Work out the finished part from the listing and answer in its coordinate system (mm). Face numbers are marked on the shaded views. A direction names the side the tool comes from. Coordinates: 2 decimals unless noted, no trailing zeros. Order: outer loops, then holes, each group sorted by start corner. A loop starts at its lowest first (then second) coordinate and runs counter-clockwise, first axis right, second up. Notation, with made-up numbers: (24.5, -13) -> (68.5, -13) arc R21 ccw to (68.5, 4) -> close; hole circle Ø3 at (-5.75, -31.75). An arc over 180 degrees is marked (long way). Use one line per item in the form item = value.
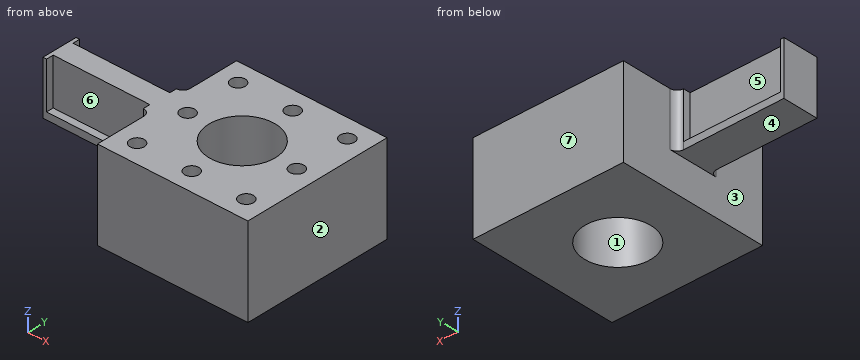
from build123d import *

# Parameters (mm, degrees)
SKETCH_1_W          = 42
SKETCH_1_H          = 42
EXTRUDE_1_DEPTH     = 25
SKETCH_2_R          = 9.25
CUT_EXTRUDE_1_DEPTH = 65.443773943
SKETCH_3_R          = 2
CUT_EXTRUDE_2_DEPTH = 3
EXTRUDE_2_DEPTH     = 30
SKETCH_5_W          = 27
SKETCH_5_H          = 13
CUT_EXTRUDE_3_DEPTH = 2
SKETCH_6_W          = 27
SKETCH_6_H          = 13
CUT_EXTRUDE_4_DEPTH = 2
FILLET_1_R          = 2


with BuildPart() as part:
    # 스케치1 → 보스-돌출1 (new body)
    with BuildSketch(Plane.XY):
        with Locations((21, -21)):
            Rectangle(SKETCH_1_W, SKETCH_1_H)
    extrude(amount=EXTRUDE_1_DEPTH)

    # 스케치2 → 컷-돌출1 (cut, through all)
    with BuildSketch(Plane.XY.offset(25)):
        with Locations((21, -21)):
            Circle(SKETCH_2_R)
    extrude(amount=-CUT_EXTRUDE_1_DEPTH, mode=Mode.SUBTRACT)

    # 스케치3 → 컷-돌출2 (cut)
    with BuildSketch(Plane.XY.offset(25)):
        with Locations((36.25, -36.25)):
            Circle(SKETCH_3_R)
        with Locations((5.75, -36.25)):
            Circle(SKETCH_3_R)
        with Locations((36.25, -5.75)):
            Circle(SKETCH_3_R)
        with Locations((5.75, -5.75)):
            Circle(SKETCH_3_R)
        with Locations((36.25, -21)):
            Circle(SKETCH_3_R)
        with Locations((21, -5.75)):
            Circle(SKETCH_3_R)
        with Locations((21, -36.25)):
            Circle(SKETCH_3_R)
        with Locations((5.75, -21)):
            Circle(SKETCH_3_R)
    extrude(amount=-CUT_EXTRUDE_2_DEPTH, mode=Mode.SUBTRACT)

    # 스케치4 → 보스-돌출2 (add)
    with BuildSketch(Plane.ZY):
        Polygon((25, -21), (25, -26), (10, -26), (10, -16), (25, -16), align=None)
    extrude(amount=EXTRUDE_2_DEPTH)

    # 스케치5 → 컷-돌출3 (cut)
    with BuildSketch(Plane(origin=(0, -26, 0), x_dir=(-1, 0, 0), z_dir=(0, -1, 0))):
        with Locations((15.5, -18.5)):
            Rectangle(SKETCH_5_W, SKETCH_5_H)
    extrude(amount=-CUT_EXTRUDE_3_DEPTH, mode=Mode.SUBTRACT)

    # 스케치6 → 컷-돌출4 (cut)
    with BuildSketch(Plane(origin=(0, -16, 0), x_dir=(1, 0, 0), z_dir=(0, 1, 0))):
        with Locations((-15.5, -18.5)):
            Rectangle(SKETCH_6_W, SKETCH_6_H)
    extrude(amount=-CUT_EXTRUDE_4_DEPTH, mode=Mode.SUBTRACT)

    # 필렛1
    fillet_1_edges = [part.edges().sort_by_distance(p)[0] for p in [
        (0, -16, 17.5),
        (0, -26, 17.5),
    ]]
    fillet(fillet_1_edges, radius=FILLET_1_R)


solid = part.part
(1) The mould has two halves that part along X. Classify the marked faces 1, 2 and 3: released by +X, released by -X, zero draft, split by the parting line, or undercut.
Data:
face_1 = undercut
face_2 = released by +X
face_3 = released by -X
(2) Section C-C on y = -5.75 is taken. Write down the section's boundary in (x, z), plus the area to 3 significant figures.
Data:
outline = (0, 0) -> (42, 0) -> (42, 25) -> (38.25, 25) -> (38.25, 22) -> (34.25, 22) -> (34.25, 25) -> (23, 25) -> (23, 22) -> (19, 22) -> (19, 25) -> (7.75, 25) -> (7.75, 22) -> (3.75, 22) -> (3.75, 25) -> (0, 25) -> close
area = 1,010 mm²
(3) Section B-B on x = 12.5 is taken. Write down the section's boundary in (y, z).
Data:
outline = (-42, 0) -> (-24.65, 0) -> (-24.65, 25) -> (-42, 25) -> close; (-17.35, 0) -> (0, 0) -> (0, 25) -> (-17.35, 25) -> close
(4) Each of these flat-tipped pins is pushed along its axis until it touches: P1, Ø7.5, axis at x = -20.5, z = 20, coming from the +Y side; P2, Ø3.5, axis at x = 21, y = -36.25, coming from the +Z side; P3, Ø4.5, axis at x = -19, z = 21, coming from the -Y side. Where does it stop, or does it pass through?
Data:
P1 = -18
P2 = 22
P3 = -24
(5) Section A-A on z = 20 is taken. Write down the section's boundary in (x, y), plus the area to 3 significant figures.
Data:
outline = (-30, -26) -> (-29, -26) -> (-29, -24) -> (-2, -24) -> (-2, -26) arc R2 cw to (0, -28) -> (0, -42) -> (42, -42) -> (42, 0) -> (0, 0) -> (0, -14) arc R2 cw to (-2, -16) -> (-2, -18) -> (-29, -18) -> (-29, -16) -> (-30, -16) -> close; hole circle Ø18.5 at (21, -21)
area = 1,690 mm²
(6) Which of the six approach directions +Z, -Z, +X, -X, +Y, -Y give full straight-line access (tool end or side, diameter ignored) to the marked faces 4, 5, 6 and 7?
Data:
face_4 = -Z, -X, +Y, -Y
face_5 = +Z, +Y
face_6 = +Z, -Y
face_7 = +Z, -Z, +X, -X, +Y
(7) Straight lines are drawn through the part: line 1 along X through (y, z) = (-36.5, 22.5); line 2 along Y through (x, z) = (5.75, 23.75); line 3 along X through (y, z) = (-38.5, 15). For each, find the intervals that lie inside material, in ascending order.
Data:
line_1 = 0 to 3.77, 7.73 to 19.02, 22.98 to 34.27, 38.23 to 42
line_2 = -42 to -38.25, -34.25 to -23, -19 to -7.75, -3.75 to 0
line_3 = 0 to 42
(8) Section D-D on x = -15.5 is taken. Write down the section's boundary in (y, z).
Data:
outline = (-26, 10) -> (-16, 10) -> (-16, 12) -> (-18, 12) -> (-18, 25) -> (-24, 25) -> (-24, 12) -> (-26, 12) -> close
